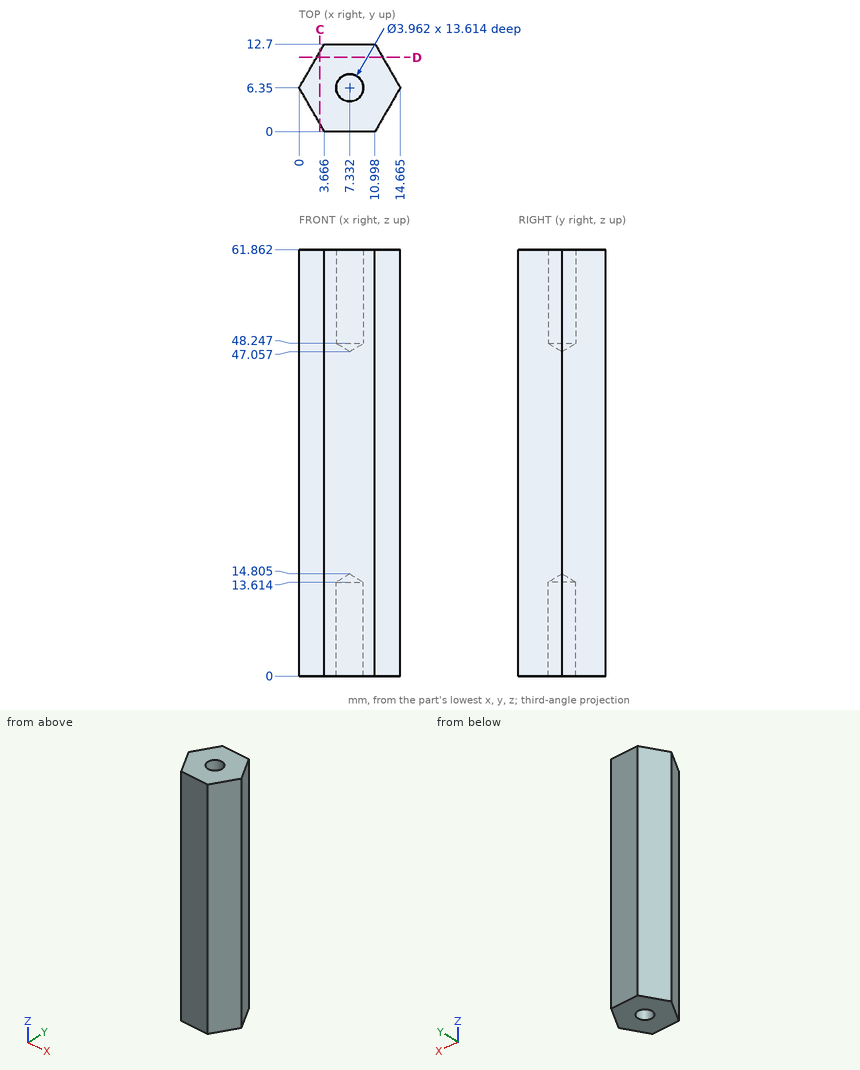
Design review of the part shown in the three views and the two pictorial views. Dimensions are in mm from the part's minimum x, y and z. Round coordinates to 2 decimals unless told otherwise and drop trailing zeros. Write each loop counter-clockwise with the first axis right and the second up, starting at its lowest first coordinate (ties: lowest second). Pieces come first, ordered by that corner, then holes.
Item 1: We need section C-C on x = 3. Write out the cut boundary in (y, z).
Item 2: Clearance check with flat-ended pins moving along their axes: pin 1 Ø6 at (y, z) = (1.5, 49.5) entering from +X; pin 2 Ø1.5 at (y, z) = (5.5, 34.5) entering from +X; pin 3 Ø3 at (x, z) = (11.5, 28.5) entering from +Y; pin 4 Ø3.5 at (x, y) = (7.33, 6.35) entering from -Z. State where each tip first meets the part, or that it passes through.
Item 3: We need section D-D on y = 10.75. Write out the cut boundary in (x, z) (1 decimal), and give its area (3 significant figures).
Item 4: For probe 1 along X at (y, z) = (7.75, 8) (1 decimal); probe 2 along Y at (x, z) = (6.5, 6.5); probe 3 along X at (y, z) = (4, 35) (1 decimal), list the stretches that pass through material, from the lowest coordinate up.
Returned:
1. outline: (1.15, 0) - (11.55, 0) - (11.55, 61.86) - (1.15, 61.86) - close
2. pin 1: stops at x = 13.6
2. pin 2: stops at x = 14.61
2. pin 3: stops at y = 12.7
2. pin 4: stops at z = 13.75
3. outline: (2.5, 0) - (12.1, 0) - (12.1, 61.9) - (2.5, 61.9) - close
3. area: 593 mm2
4. probe 1: x = 0.8 to 5.9, 8.7 to 13.9
4. probe 2: y = 0 to 4.55, 8.15 to 12.7
4. probe 3: x = 1.4 to 13.3
